Verification items for the finished model (mm, model axes). A direction names the side the tool comes from. Coordinates: 2 decimals unless noted, no trailing zeros. Write each loop counter-clockwise with the first axis right and the second up, starting at its lowest first coordinate (ties: lowest second). Pieces come first, ordered by that corner, then holes. Notation, with made-up numbers: (10.5, 41.25) -> (55.5, 41.25) arc R18 cw to (55.5, 62.25) -> close; hole circle Ø6 at (6, 70.5). An arc over 180 degrees is marked (long way). Answer in a Markdown table with one row per item.
Autodesk Fusion 360 part; units mm, degrees
sketch "スケッチ1" plane through (0, 0, 0) normal (0, 1, 0) x (1, 0, 0)
  line L0 (-20, -14) -> (-20, -41)
  line L1 (-20, -41) -> (20, -41)
  line L2 (20, -41) -> (20, -14)
  line L3 (20, -14) -> (37, -14)
  line L4 (37, -14) -> (37, 0)
  line L5 (37, 0) -> (68, 0)
  line L6 (68, 0) -> (68, -10)
  line L7 (68, -10) -> (72, -10)
  line L8 (72, -10) -> (72, -20)
  line L9 (72, -20) -> (68, -20)
  line L10 (68, -20) -> (68, -30)
  line L11 (68, -30) -> (72, -30)
  line L12 (72, -30) -> (72, -40)
  line L13 (72, -40) -> (68, -40)
  line L14 (68, -40) -> (68, -50)
  line L15 (68, -50) -> (-148, -50)
  line L16 (-148, 0) -> (-28, 0)
  line L17 (-148, 0) -> (-148, -10)
  line L18 (-148, -10) -> (-152, -10)
  line L19 (-152, -10) -> (-152, -20)
  line L20 (-152, -20) -> (-148, -20)
  line L21 (-148, -20) -> (-148, -30)
  line L22 (-148, -30) -> (-152, -30)
  line L23 (-152, -30) -> (-152, -40)
  line L24 (-152, -40) -> (-148, -40)
  line L25 (-148, -40) -> (-148, -50)
  line L26 (-108, 0) -> (-92, 0)
  line L27 (-92, 0) -> (-92, -10)
  line L28 (-92, -10) -> (-108, -10)
  line L29 (-108, -10) -> (-108, 0)
  line L30 (-68, -50) -> (-52, -50)
  line L31 (-52, -50) -> (-52, -55)
  line L32 (-52, -55) -> (-68, -55)
  line L33 (-68, -55) -> (-68, -50)
  line L34 (-138, 0) -> (-122, 0)
  line L35 (-122, 0) -> (-122, 5)
  line L36 (-122, 5) -> (-138, 5)
  line L37 (-138, 5) -> (-138, 0)
  circle A0 centre (-105, -26) radius 11.15
  line L38 (-93.9654, -24.4) -> (-93.9654, -27.6)
  line L39 (-93.9654, -27.6) -> (-91.5, -27.6)
  line L40 (-91.5, -27.6) -> (-91.5, -24.4)
  line L41 (-91.5, -24.4) -> (-93.9654, -24.4)
  line L42 (56, -50) -> (44, -50)
  line L43 (44, -50) -> (44, -42)
  line L44 (44, -42) -> (56, -42)
  line L45 (56, -42) -> (56, -50)
  line L46 (-28, 0) -> (-28, -14)
  line L47 (-28, -14) -> (-20, -14)
  point P0 (-100, 0)
  point P1 (-130, 0)
  point P2 (-60, -50)
  dimension "d8" = 20
  dimension "d9" = 20
  dimension "d10" = 14
  dimension "d11" = 68
  dimension "d12" = 4
  dimension "d13" = 10
  dimension "d14" = 10
  dimension "d15" = 10
  dimension "d16" = 10
  dimension "d17" = 10
  dimension "d19" = 17
  dimension "d34" = 4
  dimension "d37" = 216
  dimension "d40" = 100
  dimension "d41" = 10
  dimension "d42" = 16
  dimension "d43" = 5
  dimension "d44" = 16
  dimension "d45" = 60
  dimension "d46" = 130
  dimension "d49" = 22.3
  dimension "d51" = 3.2
  dimension "d52" = 105
  dimension "d53" = 26
  dimension "d54" = 13.5
  dimension "d56" = 12
  dimension "d57" = 8
  dimension "d58" = 12
  dimension "d59" = 41
  dimension "d60" = 8
extrude "押し出し1" add sketch "スケッチ1" along normal blind 4 contours L0 L1 L2 L3 L4 L5 L6 L7 L8 L9 L10 L11 L12 L13 L14 L15 L16 L17 L18 L19 L20 L21 L22 L23 L24 L25 L27 L28 L29 L30 L34 L43 L44 L45 L46 L47 | L16 L34 L35 L36 L37 | L15 L30 L31 L32 L33
sketch "スケッチ2" plane through (0, 4, 0) normal (0, 1, 0) x (-1, 0, 0)
  line L0 (-56, 50) -> (-68, 50)
  line L1 (-68, 50) -> (-68, 40)
  line L2 (-68, 40) -> (-72, 40)
  line L3 (-72, 40) -> (-72, 30)
  line L4 (-72, 30) -> (-68, 30)
  line L5 (-68, 30) -> (-68, 20)
  line L6 (-68, 20) -> (-72, 20)
  line L7 (-72, 20) -> (-72, 10)
  line L8 (-72, 10) -> (-68, 10)
  line L9 (-68, 10) -> (-68, 0)
  line L10 (-68, 0) -> (-37, 0)
  line L11 (-37, 0) -> (-37, 14)
  line L12 (-37, 14) -> (-20, 14)
  line L13 (-20, 14) -> (-20, 41)
  line L14 (-20, 41) -> (20, 41)
  line L15 (20, 41) -> (20, 14)
  line L16 (28, 0) -> (92, 0)
  line L17 (-54.5, 25) -> (-68, 25)
  line L18 (60, 36.5) -> (115, 5)
  line L19 (148, 0) -> (148, 10)
  line L20 (148, 10) -> (152, 10)
  line L21 (152, 10) -> (152, 20)
  line L22 (152, 20) -> (148, 20)
  line L23 (148, 20) -> (148, 30)
  line L24 (148, 30) -> (152, 30)
  line L25 (152, 30) -> (152, 40)
  line L26 (152, 40) -> (148, 40)
  line L27 (148, 40) -> (148, 50)
  line L28 (148, 25) -> (134.5, 25)
  line L29 (92, 0) -> (92, 10)
  line L30 (92, 10) -> (108, 10)
  line L31 (108, 10) -> (108, 0)
  line L32 (122, 0) -> (122, -5)
  line L33 (122, -5) -> (138, -5)
  line L34 (138, -5) -> (138, 0)
  line L35 (68, 50) -> (68, 55)
  line L36 (68, 55) -> (52, 55)
  line L37 (52, 55) -> (52, 50)
  line L38 (52, 50) -> (-44, 50)
  line L39 (108, 0) -> (122, 0)
  line L40 (93.9654, 24.4) -> (91.5, 24.4)
  line L41 (91.5, 24.4) -> (91.5, 27.6)
  line L42 (91.5, 27.6) -> (93.9654, 27.6)
  arc A0 (93.9654, 24.4) -> (93.9654, 27.6) centre (105, 26) ccw
  line L43 (-44, 50) -> (-44, 42)
  line L44 (-44, 42) -> (-56, 42)
  line L45 (-56, 42) -> (-56, 50)
  line L46 (148, 50) -> (68, 50)
  line L47 (20, 14) -> (28, 14)
  line L48 (28, 14) -> (28, 0)
  line L49 (138, 0) -> (148, 0)
  dimension "d24" = 13.5
  dimension "d25" = 5
  dimension "d27" = 13.5
  dimension "d38" = 60
  dimension "d39" = 115
hole "穴1" at (-115, 4, 5) at (-60, 4, 36.5) at (54.5, 4, 25) at (-134.5, 4, 25) direction (0, -1, 0) diameter 3.2 end through all
fillet "フィレット1" radius 20 2 edges at (20, 2, 41) (-20, 2, 41)
chamfer "面取り1" distance 1 angle 45 2 edges at (-122, 2, -5) (-138, 2, -5)
1. Section check C-C, the plane x = -33. Record the boundary of the cut face in (y, z).
Geometry says:
| item | result |
|---|---|
| outline | (0, 0) -> (4, 0) -> (4, 50) -> (0, 50) -> close |
2. Tool access check on faces 4 (the flat face through (68, 2, 5)), 5 (the flat face through (70, 2, 30)), 6 (the flat face through (-150, 2, 40)), 7 (the flat face through (-52, 2, 52)), 8 (the flat face through (-100, 2, 10)). Record the directions out of +Z, -Z, +X, -X, +Y, -Y that give a thin tool (end or side, any length) a straight path to the whole face; none if there is none.
Geometry says:
| item | result |
|---|---|
| face 4 | -Z, +X, +Y, -Y |
| face 5 | +X, +Y, -Y |
| face 6 | +Z, -X, +Y, -Y |
| face 7 | +Z, +X, +Y, -Y |
| face 8 | -Z, +Y, -Y |
3. Section check A-A, the plane z = 33. Record the boundary of the cut face in (x, y), plus the area to 3 significant figures.
Geometry says:
| item | result |
|---|---|
| outline | (-152, 0) -> (-113.68, 0) -> (-113.68, 4) -> (-152, 4) -> close; (-96.32, 0) -> (-16, 0) -> (-16, 4) -> (-96.32, 4) -> close; (16, 0) -> (72, 0) -> (72, 4) -> (16, 4) -> close |
| area | 699 mm^2 |
4. Section check B-B, the plane y = 0.8. State how many separate pieces and enclosed holes the cut face has, plus the area to 3 significant figures.
Geometry says:
| item | result |
|---|---|
| separate pieces | 1 |
| enclosed holes | 5 |
| area | 8,610 mm^2 |
5. Thickness scan on line 1 (X direction, y = 2.2, z = 5); line 2 (X direction, y = 3.8, z = 13.5); line 3 (X direction, y = 2.2, z = 25). Record the ranges inside material, lowest first. Write a range as from..to.
Geometry says:
| item | result |
|---|---|
| line 1 | -148..-116.6, -113.4..-108, -92..-28, 37..68 |
| line 2 | -152..-28, 37..72 |
| line 3 | -148..-136.1, -132.9..-116.11, -91.5..-19.6, 19.6..52.9, 56.1..68 |
6. Depth check by flat-ended pin: P1, Ø1.2, axis at x = -25.5, y = 1.5, coming from the -Z side; P2, Ø1.5, axis at x = 12.5, y = 0.5, coming from the -Z side; P3, Ø2, axis at y = 1.5, z = 45, coming from the +X side. Enter the tip coordinate at first touch or a pass-through.
Geometry says:
| item | result |
|---|---|
| P1 | z = 14 |
| P2 | z = 35.98 |
| P3 | x = 68 |
7. Mould release check, pull along X, two halves, no side actions. Record for faces 1 (the flat face through (28, 2, 14)), 2 (the flat face through (-122, 2, -2)), 3 (the flat face through (-150, 2, 10)): released by +X, released by -X, zero draft, split by the parting line, or undercut.
Geometry says:
| item | result |
|---|---|
| face 1 | undercut |
| face 2 | released by +X |
| face 3 | zero draft |
